Check sheet for the modelled part. Datum: model origin and axes. Units: mm. A direction names the side the tool comes from. Coordinates: 2 decimals unless noted, no trailing zeros. Loops run counter-clockwise (first coordinate to the right, second up) from the corner with the lowest first, then second, coordinate; pieces in that order, holes last. Notation, with made-up numbers: (35.5, -21) -> (83.5, -21) arc R22 ccw to (83.5, -15) -> close; hole circle Ø10 at (35.5, 45.25). An arc over 180 degrees is marked (long way). Use CSV: the item, a comma, the result in double quotes.
```python
from build123d import *

# Parameters (mm, degrees)
F1_DEPTH = 25
F2_R     = 2.5
F3_DEPTH = 25


with BuildPart() as f1:
    # F0 (on Front) → F1 (new body)
    with BuildSketch(Plane.XZ):
        Polygon((15.035118, 20.081509), (-32.964882, 20.081509), (-32.964882, -29.918491), (-29.964882, -29.918491), (-29.964882, 17.081509), (15.035118, 17.081509), align=None)
    extrude(amount=F1_DEPTH)

    # F2 (on face) → F3 (cut)
    with BuildSketch(Plane(origin=(-32.964882, 0, 0), x_dir=(0, -1, 0), z_dir=(-1, 0, 0))):
        with Locations((22.227423, 0.081509)):
            Circle(F2_R)
        with Locations((4.864288, 0.081509)):
            Circle(F2_R)
    extrude(amount=-F3_DEPTH, mode=Mode.SUBTRACT)


solid = f1.part
```
1) Cross-section at C-C on x = 8. Record the boundary of the cut face in (y, z).
Answer below:
outline,"(-25, 17.08) -> (0, 17.08) -> (0, 20.08) -> (-25, 20.08) -> close"
2) Thickness scan on line 1 along Z through (x, y) = (-23, -12.5); line 2 along X through (y, z) = (-20.25, -16.5). Record the ranges inside material, lowest first. Write a range as from..to.
Answer below:
line 1,"z = 17.08..20.08"
line 2,"x = -32.96..-29.96"
3) Cross-section at B-B on y = -20.5. Record the boundary of the cut face in (x, z).
Answer below:
outline,"(-32.96, -29.92) -> (-29.96, -29.92) -> (-29.96, -1.73) -> (-32.96, -1.73) -> close; (-32.96, 1.89) -> (-29.96, 1.89) -> (-29.96, 17.08) -> (15.04, 17.08) -> (15.04, 20.08) -> (-32.96, 20.08) -> close"
4) Access from +Z, -Z, +X, -X, +Y, -Y to the whole of each face (thin tool, end or side, straight path). Record for faces 1 (the cylindrical face through (-31.49, -7.25, 0.83)), 2 (the flat face through (-29.965, -12, -7)).
Answer below:
face 1,"+X, -X"
face 2,"-Z, +X, +Y, -Y"
5) Go/stop test with flat-tipped pins: pin 1 Ø3 at (x, y) = (4, -18.5) entering from -Z; pin 2 Ø6 at (y, z) = (-15.5, -10) entering from +X. Record where each tip stops, or that it passes through.
Answer below:
pin 1,"stops at z = 17.08"
pin 2,"stops at x = -29.96"
6) Cross-section at A-A on z = -1. Record the boundary of the cut face in (x, y), and give its area (3 significant figures).
Answer below:
outline,"(-32.96, -25) -> (-29.96, -25) -> (-29.96, -24.48) -> (-32.96, -24.48) -> close; (-32.96, -19.97) -> (-29.96, -19.97) -> (-29.96, -7.12) -> (-32.96, -7.12) -> close; (-32.96, -2.61) -> (-29.96, -2.61) -> (-29.96, 0) -> (-32.96, 0) -> close"
area,"48.0 mm²"
7) Cross-section at D-D on y = -17.25. Record the boundary of the cut face in (x, z).
Answer below:
outline,"(-32.96, -29.92) -> (-29.96, -29.92) -> (-29.96, 17.08) -> (15.04, 17.08) -> (15.04, 20.08) -> (-32.96, 20.08) -> close"
